Check sheet for the modelled part. Datum: model origin and axes. Units: mm. A direction names the side the tool comes from. Round coordinates to 2 decimals unless told otherwise and drop trailing zeros. Order: outer loops, then holes, each group sorted by start corner. A loop starts at its lowest first (then second) coordinate and runs counter-clockwise, first axis right, second up. Notation, with made-up numbers: (71.5, -28.75) -> (81.5, -28.75) arc R10 cw to (81.5, -10.75) -> close; hole circle Ø8 at (75.5, 54.5). An arc over 180 degrees is marked (long way). Answer in a Markdown table with one row per item.
Autodesk Inventor part; units mm, degrees
ref_plane "PoleBase Plane" through (57.325, 9.4828, 4.9562) normal (0, 0.9996, -0.03) x (-1, 0, 0)
ref_plane "YZ Plane" through (0, 0, 0) normal (1, 0, 0) x (0, 1, 0)
ref_plane "XZ Plane" through (0, 0, 0) normal (0, 1, 0) x (-1, 0, 0)
sketch "Spacebar base" plane through (0, 0, 0) normal (0, 1, 0) x (-1, 0, 0)
  line L0 (58.825, 9.05) -> (-58.825, 9.05)
  line L1 (-58.825, 9.05) -> (-58.825, -9.05)
  line L2 (-58.825, -9.05) -> (58.825, -9.05)
  line L3 (58.825, -9.05) -> (58.825, 9.05)
  line L4 (58.825, 9.05) -> (-58.825, -9.05) construction
  line L5 (-58.825, 9.05) -> (58.825, -9.05) construction
  point P0 (0, 0)
  dimension "d0" = 117.65
  dimension "d1" = 18.1
extrude "Spacebar Bulk" add sketch "Spacebar base" along normal blind 11
sketch "Curve Profile" plane through (58.825, 0, 9.05) normal (1, 0, 0) x (0, 0, -1)
  line L0 (0, 0) -> (18.1, 0)
  line L1 (0, 0) -> (2.9474, 11)
  line L2 (0, 11) -> (18.1, 11)
  line L3 (18.1, 0) -> (18.1, 11)
  arc A0 (18.1, 8) -> (2.9474, 11) centre (2.9474, -28.7667) ccw
  line L4 (0, 0) -> (0, 11)
  line L5 (18.1, 8) -> (18.1, 0)
  line L6 (18.1, 0) -> (0, 0)
  point P0 (9.05, 0)
  dimension "d4" = 15
  dimension "d9" = 8
extrude "Curve Cutaway" cut sketch "Curve Profile" against normal up to surface (117.65 mm away) contours L1 A0 L3 L0 keep common part
shell "Inner Shell" thickness 1.5 removed faces 1 at (19.6083, 0, 3.0167)
ref_plane "PoleBase Plane" through (57.325, 9.4828, 4.9562) normal (0, 0.9996, -0.03) x (-1, 0, 0)
sketch "Center Circle" plane through (57.325, 9.4828, 4.9562) normal (0, 0.9996, -0.03) x (-1, 0, 0)
  circle A0 centre (57.325, -5.238) radius 2.77
  dimension "d11" = 5.54
extrude "Pole Extrusion" add sketch "Center Circle" against normal up to surface surface through (0, 0, 0) normal (0, 1, 0)
sketch "Sketch4" plane through (0, 0, 0) normal (0, -1, 0) x (1, 0, 0)
  line L0 (-2.175, 0.8) -> (2.175, 0.8)
  line L1 (2.175, 0.8) -> (2.175, -0.8)
  line L2 (2.175, -0.8) -> (-2.175, -0.8)
  line L3 (-2.175, -0.8) -> (-2.175, 0.8)
  line L4 (-2.175, 0.8) -> (2.175, -0.8) construction
  line L5 (2.175, 0.8) -> (-2.175, -0.8) construction
  line L6 (0.8, 2.175) -> (-0.8, 2.175)
  line L7 (-0.8, 2.175) -> (-0.8, -2.175)
  line L8 (-0.8, -2.175) -> (0.8, -2.175)
  line L9 (0.8, -2.175) -> (0.8, 2.175)
  line L10 (0.8, 2.175) -> (-0.8, -2.175) construction
  line L11 (-0.8, 2.175) -> (0.8, -2.175) construction
  point P0 (0, 0)
  dimension "d14" = 4.35
  dimension "d15" = 1.6
  dimension "d16" = 1.6
  dimension "d17" = 4.35
extrude "Extrusion4" cut sketch "Sketch4" against normal blind 5
equation "\"d0\" = b_space"
equation "\"d1\" = k_width"
equation "\"d10\" = k_wthick"
equation "\"d11\" = k_poledia"
equation "\"d14\" = k_cmxl"
equation "\"d15\" = k_cmxw"
equation "\"d16\" = k_cmxw"
equation "\"d17\" = k_cmxl"
equation "\"k_width\" = 18.1"
equation "\"k_height\" = 18"
equation "\"k_height_t\" = 16"
equation "\"k_taper1\" = 1.5"
equation "\"k_taper2\" = 0.5"
equation "\"k_staper\" = 1"
equation "\"k_sradius\" = 4"
equation "\"k_ltaper\" = 1.5"
equation "\"k_lradius\" = 6"
equation "\"k_radius\" = 6"
equation "\"k_wthick\" = 1.5"
equation "\"k_ribthick\" = 1.5"
equation "\"k_ribheight\" = 5"
equation "\"k_poleoff\" = 2.2625"
equation "\"k_poledia\" = 5.54"
equation "\"k_cmxw\" = 1.6"
equation "\"k_cmxl\" = 4.35"
equation "\"s_bwidth\" = 15.6"
equation "\"s_poleh\" = 3.6"
equation "\"s_polebw\" = 5.5"
equation "\"s_polebl\" = 7"
equation "\"b_pad\" = 1"
equation "\"b_tab\" = 27.15"
equation "\"b_caps\" = 31.675"
equation "\"b_lshift\" = 40.725"
equation "\"b_rshift\" = 49.775"
equation "\"b_ctrl\" = 22.625"
equation "\"b_space\" = 117.65"
equation "\"b_width\" = 286.5"
equation "\"b_height\" = 77.4"
equation "\"k_taper_wide\" = 1.5"
equation "\"k_height_low\" = 16"
equation "\"k_taper_thin\" = 0.5"
properties part number "spacebar-keycap_mockup_cherrymx"
Item 1: Cross-section at C-C (y = 3). State how many separate pieces and enclosed holes the cut face has, and give its area (3 significant figures).
Result sheet:
| item | result |
|---|---|
| separate pieces | 2 |
| enclosed holes | 2 |
| area | 415 mm^2 |
Item 2: Mould release check, pull along X, two halves, no side actions. Record for faces 4 (the flat face through (0.824, 5.423, 7.597)), 5 (the flat face through (58.825, 5, 0)), 6 (the flat face through (-58.825, 5, 0)), 7 (the flat face through (0.803, 4.675, 6.244)): pulls with the +X half, pulls with the -X half, needs draft (parallel to the pull), parting line crosses it, or undercut.
Result sheet:
| item | result |
|---|---|
| face 4 | needs draft |
| face 5 | pulls with the +X half |
| face 6 | pulls with the -X half |
| face 7 | undercut |
Item 3: Depth check by flat-ended pin: P1, Ø0.8, axis at x = 0, y = 3, coming from the +Z side; P2, Ø1.1, axis at x = 1, y = 3.5, coming from the +Z side; P3, Ø1, axis at x = 35.5, z = -7, coming from the +Y side. Enter the tip coordinate at first touch or a pass-through.
Result sheet:
| item | result |
|---|---|
| P1 | stops at z = 8.35 |
| P2 | stops at z = 8.26 |
| P3 | stops at y = 8.95 |
Item 4: Cross-section at A-A (x = -6). Record the boundary of the cut face in (y, z).
Result sheet:
| item | result |
|---|---|
| outline | (0, -9.05) -> (8, -9.05) arc R39.77 ccw to (11, 6.1) -> (0, 9.05) -> (0, 7.5) -> (9.48, 4.96) arc R38.27 cw to (6.98, -7.55) -> (0, -7.55) -> close |
Item 5: Set-up check for faces 1 (the flat face through (1, 4, -9.05)), 2 (the flat face through (-57.325, 5, 0)), 3 (the cylindrical face through (-1.489, 4.717, 2.196)): record each of +Z, -Z, +X, -X, +Y, -Y from which the full face is reachable in a straight line by a thin tool's end or side.
Result sheet:
| item | result |
|---|---|
| face 1 | -Z, +X, -X, +Y, -Y |
| face 2 | -Y |
| face 3 | none |
Item 6: Cross-section at B-B (z = -4.75). Record the boundary of the cut face in (x, y) (1 decimal).
Result sheet:
| item | result |
|---|---|
| outline | (-58.8, 0) -> (-57.3, 0) -> (-57.3, 7.9) -> (57.3, 7.9) -> (57.3, 0) -> (58.8, 0) -> (58.8, 9.5) -> (-58.8, 9.5) -> close |
Item 7: Scan lines: line 1 (X direction, y = 7.75, z = 1.5) (3 decimals); line 2 (X direction, y = 6, z = -5) (3 decimals); line 3 (X direction, y = 3.5, z = 1.25) (3 decimals). Record each from-to range of solid material in increasing order. Write a range as [from, to].
Result sheet:
| item | result |
|---|---|
| line 1 | x = [-58.825, -57.325], [-2.162, 2.162], [57.325, 58.825] |
| line 2 | x = [-58.825, -57.325], [57.325, 58.825] |
| line 3 | x = [-58.825, -57.325], [-2.417, -0.8], [0.8, 2.417], [57.325, 58.825] |
